For this review, take the finished solid that the model builds, in its own axes (mm). Round coordinates to 2 decimals unless told otherwise and drop trailing zeros. Order: outer loops, then holes, each group sorted by start corner. A loop starts at its lowest first (then second) coordinate and runs counter-clockwise, first axis right, second up. Notation, with made-up numbers: (63, 29) - (87, 29) arc R21 ccw to (87, 33) - close; hole circle Ø10 at (3, 74.25). An arc over 180 degrees is marked (long way). One line per question, with ' | ' between items.
```python
from build123d import *

# Parameters (mm, degrees)
F1_DEPTH  = 3.4
F2_R      = 1.6
F2_W      = 2
F2_H      = 5
F3_DEPTH  = 9.4
F4_DEPTH  = 44.24
F5_W      = 43.4320680797
F5_H      = 5.540763028
F6_DEPTH  = 55
F7_W      = 42
F7_H      = 6
F8_DEPTH  = 25
F9_D      = 3.4
F11_DEPTH = 25


# Not quite as in the source:
# - after a boolean that leaves OpenCascade's solid faulty, fix() repairs it
# - a feature names something its author has since deleted; it is built from what else it names


with BuildPart() as f1:
    # F0 (on Right) → F1 (new body)
    with BuildSketch(Plane.YZ):
        Polygon((0, 4), (-2, 4), (-2, -4), (0, -4), (2, -4), (2, 4), align=None)
        with BuildLine():
            ThreePointArc((1.7, -2.1), (1.202081528, -3.302081528), (0, -3.8))
            ThreePointArc((0, -3.8), (-1.202081528, -0.897918472), (1.7, -2.1))
        make_face(mode=Mode.SUBTRACT)
        Polygon((-2, 8), (-2, 4), (0, 4), (2, 4), (2, 8), align=None)
        with BuildLine():
            ThreePointArc((1.7, 5.9), (1.202081528, 4.697918472), (0, 4.2))
            ThreePointArc((0, 4.2), (-1.202081528, 7.102081528), (1.7, 5.9))
        make_face(mode=Mode.SUBTRACT)
    extrude(amount=F1_DEPTH)

    # F2 (on Top) → F3 (join)
    with BuildSketch(Plane.XY):
        with BuildLine():
            Line((-42, -2.019777894), (0, -2.019777894))
            Line((0, -2.019777894), (0, 1.980222106))
            Line((0, 1.980222106), (0, 46.980222106))
            Line((0, 46.980222106), (-2, 46.980222106))
            Line((-2, 46.980222106), (-2.1, 46.980222106))
            ThreePointArc((-2.1, 46.980222106), (-3.7, 45.380222106), (-5.3, 46.980222106))
            ThreePointArc((-5.3, 46.980222106), (-4.8313708499, 48.1115929559), (-3.7, 48.580222106))
            Line((-3.7, 48.580222106), (-3.7, 51.980222106))
            Line((-3.7, 51.980222106), (-42, 51.980222106))
            Line((-42, 51.980222106), (-42, 1.980222106))
            Line((-42, 1.980222106), (-42, -2.019777894))
        make_face()
        with Locations((-33.7, 46.980222106)):
            Circle(F2_R, mode=Mode.SUBTRACT)
        with BuildLine():
            Line((-2.1, 46.980222106), (-2, 46.980222106))
            Line((-2, 46.980222106), (-2, 51.980222106))
            Line((-2, 51.980222106), (-3.7, 51.980222106))
            Line((-3.7, 51.980222106), (-3.7, 48.580222106))
            ThreePointArc((-3.7, 48.580222106), (-2.5686291501, 48.1115929559), (-2.1, 46.980222106))
        make_face()
        with Locations((-1, 49.480222106)):
            Rectangle(F2_W, F2_H)
    extrude(amount=F3_DEPTH)

    # F0 (on Right) → F4 (join)
    with BuildSketch(Plane.YZ):
        Polygon((0, 4), (-2, 4), (-2, -4), (0, -4), (2, -4), (2, 4), align=None)
        with BuildLine():
            ThreePointArc((1.7, -2.1), (1.202081528, -3.302081528), (0, -3.8))
            ThreePointArc((0, -3.8), (-1.202081528, -0.897918472), (1.7, -2.1))
        make_face(mode=Mode.SUBTRACT)
        Polygon((-2, 8), (-2, 4), (0, 4), (2, 4), (2, 8), align=None)
        with BuildLine():
            ThreePointArc((1.7, 5.9), (1.202081528, 4.697918472), (0, 4.2))
            ThreePointArc((0, 4.2), (-1.202081528, 7.102081528), (1.7, 5.9))
        make_face(mode=Mode.SUBTRACT)
    extrude(amount=-F4_DEPTH)

    # F5 (on Front) → F6 (cut)
    with BuildSketch(Plane.XZ):
        with Locations((-21.7160340399, 2.770381514)):
            Rectangle(F5_W, F5_H)
    extrude(amount=-F6_DEPTH, mode=Mode.SUBTRACT)

    # F7 (on face) → F8 (cut)
    with BuildSketch(Plane.XZ.offset(2.019777894)):
        with Locations((-21, 3)):
            Rectangle(F7_W, F7_H)
    extrude(amount=-F8_DEPTH, mode=Mode.SUBTRACT)

    # F9 (through all)
    with Locations(Plane.YZ):
        with Locations((0, 5.9)):
            Hole(F9_D / 2)

    # F10 (on face) → F11 (cut)
    with BuildSketch(Plane.XZ.offset(2)):
        Polygon((0, -4), (0, 0), (-42, 0), (-42.0278720558, -4), align=None)
    extrude(amount=-F11_DEPTH, mode=Mode.SUBTRACT)

    add(f1.part.fix(), mode=Mode.REPLACE)


solid = f1.part
```
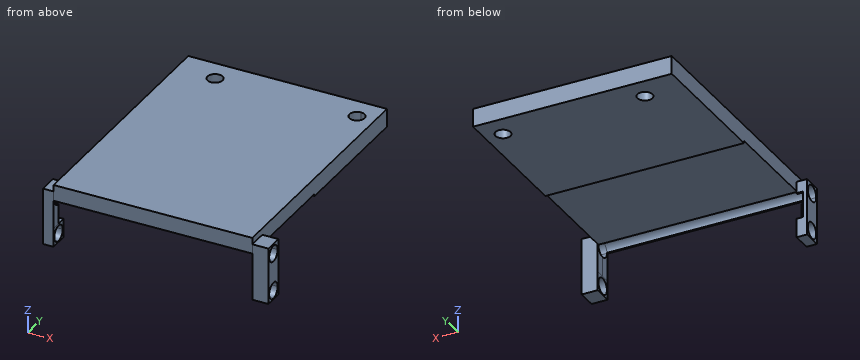
(1) Insertion check: pin 1 (1 mm diameter, centred on x = -23.5, y = 30.5, fed in from -Z); pin 2 (5 mm diameter, centred on y = 21.5, z = 5, fed in from -X); pin 3 (10.5 mm diameter, centred on x = -14, y = 16.5, fed in from -Z); pin 4 (1 mm diameter, centred on y = 14, z = 4.5, fed in from -X). Each pin has a flat end and moves straight along its axis. Give the tip position at first contact, or say it passes through.
Output values:
pin 1: z = 5.54 | pin 2: x = -42 | pin 3: z = 6 | pin 4: through
(2) We need section C-C on x = -8.5. State the section outline as (y, z) points, plus the area to 3 significant figures.
Output values:
outline: (-2.02, 6) - (-1.7, 6) arc R1.7 cw to (1.7, 6) - (22.98, 6) - (22.98, 5.54) - (51.98, 5.54) - (51.98, 9.4) - (-2.02, 9.4) - close | area: 193 mm^2
(3) We need section B-B on y = 5. State the section outline as (x, z) points, plus the area to 3 significant figures.
Output values:
outline: (-42, 6) - (0, 6) - (0, 9.4) - (-42, 9.4) - close | area: 143 mm^2
(4) For probe 1 along X at (y, z) = (47, 6.5); probe 2 along Z at (x, y) = (-5, 40.5); probe 3 along X at (y, z) = (37, 6.75), list the stretches that pass through material, from the lowest coordinate up. Write a range as [from, to].
Output values:
probe 1: [-42, -35.3], [-32.1, -5.3], [-2.1, 0] | probe 2: [5.54, 9.4] | probe 3: [-42, 0]
(5) We need section D-D on y = 36. State the section outline as (x, z) points, plus the area to 3 significant figures.
Output values:
outline: (-42, 5.54) - (0, 5.54) - (0, 9.4) - (-42, 9.4) - close | area: 162 mm^2
(6) We need section A-A on x = -33.7. State the section outline as (y, z) points, plus the area to 3 significant figures.
Output values:
outline: (-2.02, 6) - (-1.7, 6) arc R1.7 cw to (1.7, 6) - (22.98, 6) - (22.98, 5.54) - (45.38, 5.54) - (45.38, 9.4) - (-2.02, 9.4) - close; (48.58, 5.54) - (51.98, 5.54) - (51.98, 9.4) - (48.58, 9.4) - close | area: 180 mm^2
